For this review, take the finished solid that the model builds, in its own axes (mm). A direction names the side the tool comes from. Give positions to 0.01 mm unless a question says otherwise; leave off trailing zeros. Loops run counter-clockwise (first coordinate to the right, second up) from the corner with the lowest first, then second, coordinate; pieces in that order, holes last. Notation, with made-up numbers: (16.5, 45) - (23.5, 45) arc R22 ccw to (23.5, 51) - close; hole circle Ø8 at (-24.5, 15). An arc over 180 degrees is marked (long way). Put each result on its own line as item: value.
from build123d import *

# Parameters (mm, degrees)
SKETCH1_R           = 5
BOSS_EXTRUDE1_DEPTH = 6
SKETCH4_R           = 2.5
BOSS_EXTRUDE2_DEPTH = 10


with BuildPart() as part:
    # Sketch1 → Boss-Extrude1 (new body)
    with BuildSketch(Plane.XY):
        Circle(SKETCH1_R)
    extrude(amount=BOSS_EXTRUDE1_DEPTH)

    # Sketch3 → Cut-Revolve1 (revolve, cut)
    with BuildSketch(Plane(origin=(0, 0, 0), x_dir=(0, 0, -1), z_dir=(1, 0, 0)), mode=Mode.PRIVATE) as cut_revolve1_sk:
        with BuildLine():
            Line((-6, 0), (-9.957172865, 0))
            Line((-9.957172865, 0), (-9.957172865, 5.514350083))
            Line((-9.957172865, 5.514350083), (-9.957172865, 6))
            Line((-9.957172865, 6), (-6, 6))
            ThreePointArc((-6, 6), (-2.757359313, 3.828427125), (-2, 0))
            Line((-2, 0), (-6, 0))
        make_face()
    revolve(cut_revolve1_sk.sketch.rotate(Axis((0, 0, 0), (0, 0, 1)), 270), axis=Axis((0, 0, 0), (0, 0, 1)), mode=Mode.SUBTRACT)

    # Sketch4 → Boss-Extrude2 (add)
    with BuildSketch(Plane(origin=(0, 0, 0), x_dir=(-1, 0, 0), z_dir=(0, 0, -1))):
        with Locations(Location((0, 0, 0), (0, 0, 180))):
            Circle(SKETCH4_R)
    extrude(amount=BOSS_EXTRUDE2_DEPTH)


solid = part.part
1) For faces 1 (the face through (-2.5, -0.1, -4.9)), 2 (the face through (-1.08, -4.88, 1.89)), list the 3-axis set-ups (+Z, -Z, +X, -X, +Y, -Y) from which the entire face can be reached by the end or side of a thin tool; tool diameter is ignored.
Geometry check:
face 1: -Z
face 2: +Z, -Z
2) Take a section at A-A on z = -7. State the section outline as (x, y) points, and give its area (3 significant figures).
Geometry check:
outline: circle Ø5 at (0, 0)
area: 19.6 mm²
3) Insertion check: pin 1 Ø6 at (y, z) = (-2.5, -8) entering from -X; pin 2 Ø4 at (x, z) = (-3, -5) entering from +Y; pin 3 Ø1 at (y, z) = (2, 0.5) entering from +X. Each pin has a flat end and moves straight along its axis. Give the tip position at first contact, or say it passes through.
Geometry check:
pin 1: stops at x = -2.5
pin 2: stops at y = 2.29
pin 3: stops at x = 4.77
4) Wall thickness on line 1 (Y direction, x = 0.75, z = 3); line 2 (Z direction, x = 0, y = -3.5); line 3 (X direction, y = -0.75, z = -4.75): over which ranges is each line inside the solid? List them lowest first.
Geometry check:
line 1: y = -4.94 to -4.09, 4.09 to 4.94
line 2: z = 0 to 2.56
line 3: x = -2.38 to 2.38
